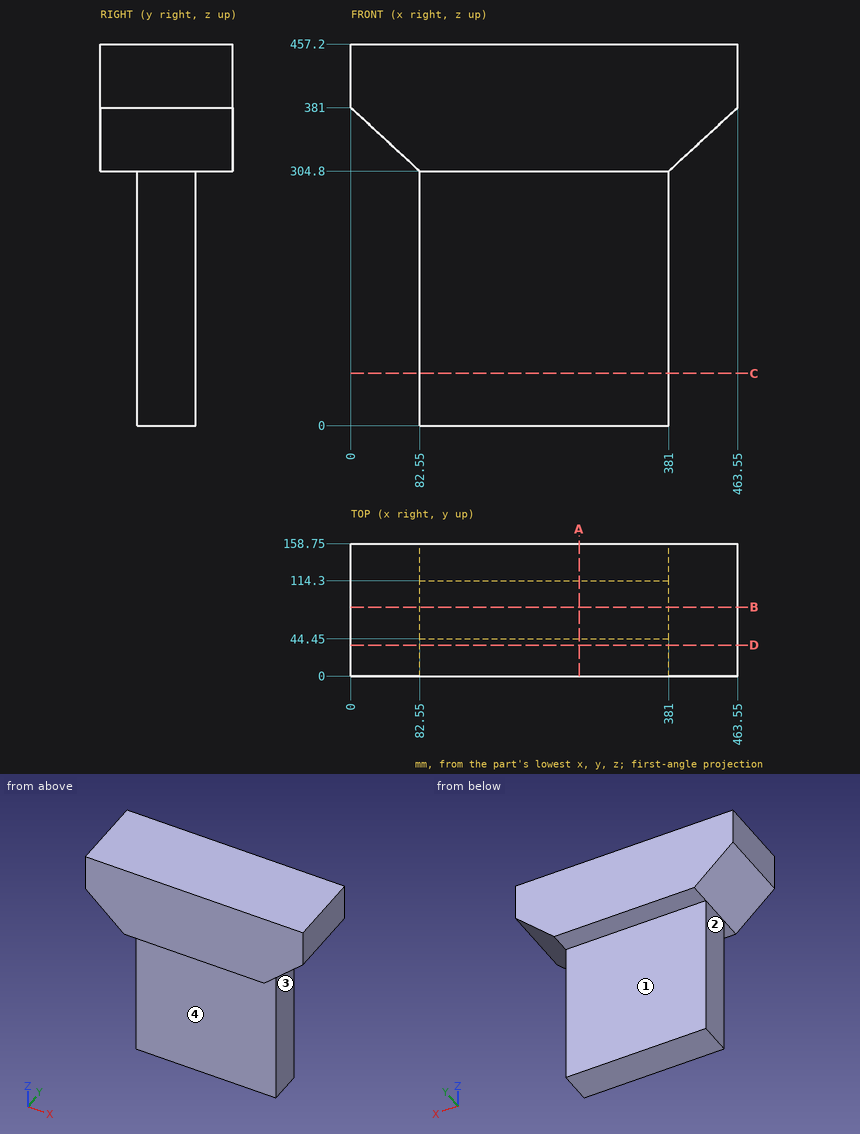
Can you work these out from the drawing? Everything is in mm from the part's minimum corner. A direction names the side the tool comes from. Round coordinates to 2 decimals unless told otherwise and drop trailing zeros. Write each loop counter-clockwise with the first axis right and the second up, starting at its lowest first coordinate (ties: lowest second). Pieces come first, ordered by that corner, then holes.
1. Suppose I cut it at A-A (x = 273.5). List the corners of the cut face in (y, z) for me.
2. Will these pins go through, and if not, where does the flat tip stop? pin 1 Ø4 at (x, z) = (313.5, 89.5) entering from +Y; pin 2 Ø13.5 at (x, y) = (239, 137) entering from -Z; pin 3 Ø4 at (y, z) = (82, 256) entering from +X.
3. Suppose I cut it at C-C (z = 62.5). List the corners of the cut face in (x, y) for me.
4. Suppose I cut it at D-D (y = 37). List the corners of the cut face in (x, z) for me.
5. For the marked faces 1, 2, 3 and 4, which set-ups out of +Z, -Z, +X, -X, +Y, -Y let a thin tool reach every point of the face, with its end or its side?
6. Suppose I cut it at B-B (y = 82.5). List the corners of the cut face in (x, z) for me.
7. I need wall thicknesses on L1, parallel to Y at x = 270.5, z = 189; L2, parallel to X at y = 55.5, z = 125.5; L3, parallel to Z at x = 242, y = 120. Which ranges of each line are inside material? Lowest first, please.
Answer sheet:
1. outline: (0, 304.8) - (44.45, 304.8) - (44.45, 0) - (114.3, 0) - (114.3, 304.8) - (158.75, 304.8) - (158.75, 457.2) - (0, 457.2) - close
2. pin 1: stops at y = 114.3
2. pin 2: stops at z = 304.8
2. pin 3: stops at x = 381
3. outline: (82.55, 44.45) - (381, 44.45) - (381, 114.3) - (82.55, 114.3) - close
4. outline: (0, 381) - (82.55, 304.8) - (381, 304.8) - (463.55, 381) - (463.55, 457.2) - (0, 457.2) - close
5. face 1: -Z, +X, -X, +Y
5. face 2: -Z, -X, +Y, -Y
5. face 3: -Z, +X, +Y, -Y
5. face 4: -Z, +X, -X, -Y
6. outline: (0, 381) - (82.55, 304.8) - (82.55, 0) - (381, 0) - (381, 304.8) - (463.55, 381) - (463.55, 457.2) - (0, 457.2) - close
7. L1: y = 44.45 to 114.3
7. L2: x = 82.55 to 381
7. L3: z = 304.8 to 457.2
